Study the drawing (mm; zero at the part's minimum x, y, z) and answer. A direction names the side the tool comes from. Give positions to 0.01 mm unless a question says otherwise; leave off trailing zeros. Order: outer loops, then holes, each group sorted by start corner. A loop starts at its lowest first (then second) coordinate and runs counter-clockwise, first axis right, second up.
Item 1: A cutting plane is placed at B-B (x = 12.5). Write down the section's boundary in (y, z).
Item 2: A cutting plane is placed at C-C (z = 62.5). Write down the section's boundary in (x, y), plus the area to 3 significant figures.
Item 3: The mould has two halves that part along X. Classify the marked faces 3, 4 and 5: +X half, -X half, draft (parallel to the pull), parting line (faces both ways), or undercut.
Item 4: Given pin 1 Ø6 at (x, z) = (20, 62.5) entering from +Y; pin 2 Ø3 at (y, z) = (36, 48) entering from +X (3 decimals); pin 3 Ø4 at (x, z) = (7, 19) entering from +Y, each flat-ended and moving along its own axis, determine where each tip first touches the part or whether it passes through.
Item 5: Find the intervals of material crossed by line 1 along X through (y, z) = (16, 30); line 2 along X through (y, z) = (31.5, 19); line 3 along Y through (x, z) = (26, 28), in increasing order.
Item 6: Which of the six approach directions +Z, -Z, +X, -X, +Y, -Y give full straight-line access (tool end or side, diameter ignored) to the marked faces 1 and 2?
Item 7: A cutting plane is placed at A-A (y = 16). Write down the section's boundary in (x, z), plus the area to 3 significant figures.
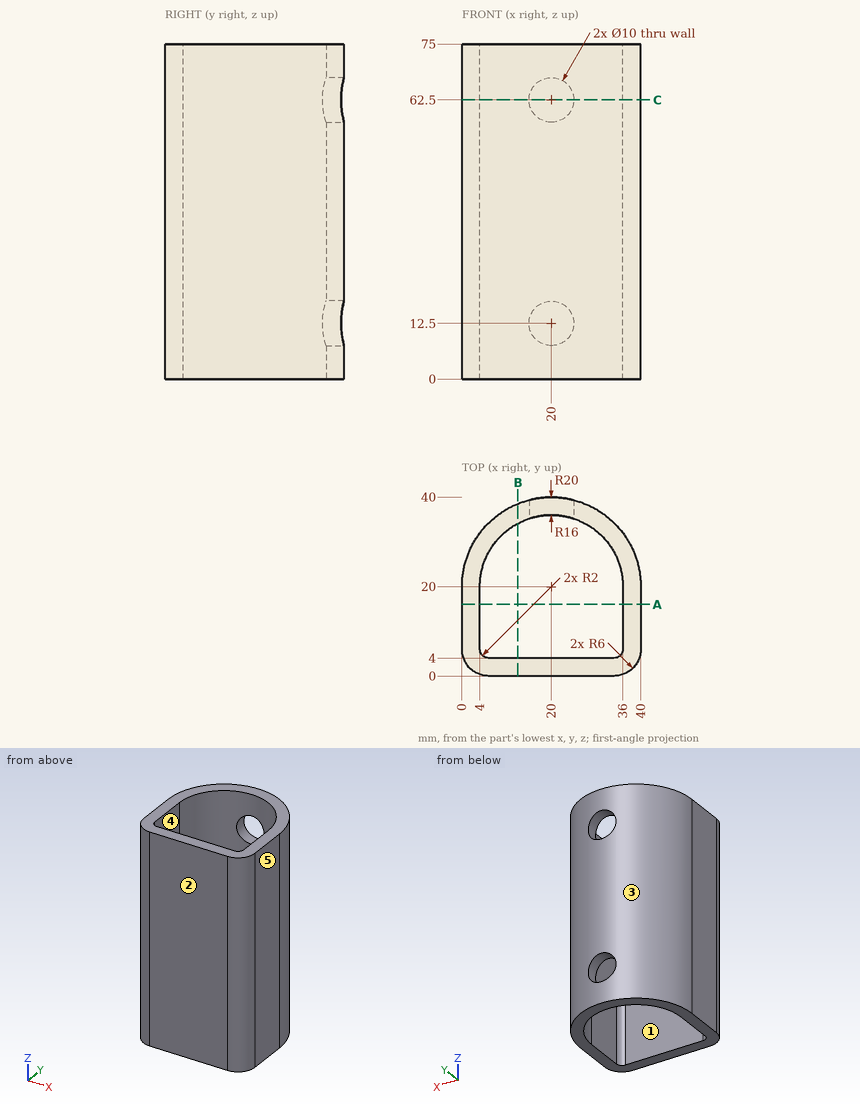
Response values:
1. outline: (0, 0) - (4, 0) - (4, 75) - (0, 75) - close; (34.13, 0) - (38.54, 0) - (38.54, 75) - (34.13, 75) - close
2. outline: (0, 6) arc R6 ccw to (6, 0) - (34, 0) arc R6 ccw to (40, 6) - (40, 20) arc R20 ccw to (25, 39.36) - (25, 35.2) arc R16 cw to (36, 20) - (36, 6) arc R2 cw to (34, 4) - (6, 4) arc R2 cw to (4, 6) - (4, 20) arc R16 cw to (15, 35.2) - (15, 39.36) arc R20 ccw to (0, 20) - close
2. area: 460 mm2
3. face 3: parting line
3. face 4: undercut
3. face 5: +X half
4. pin 1: stops at y = 4
4. pin 2: stops at x = 33.775
4. pin 3: stops at y = 36.7
5. line 1: x = 0 to 4, 36 to 40
5. line 2: x = 3.64 to 8.88, 31.12 to 36.36
5. line 3: y = 0 to 4, 34.83 to 39.08
6. face 1: +Z, -Z
6. face 2: +Z, -Z, +X, -X, -Y
7. outline: (0, 0) - (4, 0) - (4, 75) - (0, 75) - close; (36, 0) - (40, 0) - (40, 75) - (36, 75) - close
7. area: 600 mm2
